```python
from build123d import *

# Parameters (mm, degrees)
F0_R     = 4
F1_DEPTH = 2.5


with BuildPart() as f1:
    # F0 (on Front) → F1 (new body, symmetric)
    with BuildSketch(Plane.XZ):
        with BuildLine():
            Line((0, 8.455922), (-25, 8.455922))
            ThreePointArc((-25, 8.455922), (-33, 0.455922), (-25, -7.544078))
            Line((-25, -7.544078), (0, -7.544078))
            Line((0, -7.544078), (0, 8.455922))
        make_face()
        with Locations((-25, 0.455922)):
            Circle(F0_R, mode=Mode.SUBTRACT)
    extrude(amount=F1_DEPTH, both=True)

    # F2: F1 across face


with BuildPart() as f1_1:
    add(f1.part)
    add(f1.part.mirror(Plane(origin=(0, 0, 0.455922), x_dir=(0, 1, 0), z_dir=(1, 0, 0))))


solid = f1_1.part
```
Source: CAD feature listing. Evaluate the final solid. Frame: model axes, mm. Round coordinates to 2 decimals unless told otherwise and drop trailing zeros. Loops run counter-clockwise (first coordinate to the right, second up) from the corner with the lowest first, then second, coordinate; pieces in that order, holes last. Notation, with made-up numbers: M 82.25,-23.75 L 130.25,-23.75 A14 cw 130.25,-16.75 Z; hole C 42,87 d1. An arc over 180 degrees is marked long. Put each result on its own line as item: value.
(1) Section B-B, the plane z = 3. Return loops of the section in (x, y).
Solutions:
outline: M -32.58,-2.5 L -28.09,-2.5 L -28.09,2.5 L -32.58,2.5 Z; M -21.91,-2.5 L 21.91,-2.5 L 21.91,2.5 L -21.91,2.5 Z; M 28.09,-2.5 L 32.58,-2.5 L 32.58,2.5 L 28.09,2.5 Z
(2) Section D-D, the plane z = -5.75. Return loops of the section in (x, y), and give its area (3 significant figures).
Solutions:
outline: M -30.05,-2.5 L 30.05,-2.5 L 30.05,2.5 L -30.05,2.5 Z
area: 300 mm²
(3) Section A-A, the plane x = -22.5. Return loops of the section in (y, z).
Solutions:
outline: M -2.5,-7.54 L 2.5,-7.54 L 2.5,-2.67 L -2.5,-2.67 Z; M -2.5,3.58 L 2.5,3.58 L 2.5,8.46 L -2.5,8.46 Z
(4) Section C-C, the plane y = -0.7. Return loops of the section in (x, z), and give its area (3 significant figures).
Solutions:
outline: M -25,-7.54 L 25,-7.54 A8 ccw 25,8.46 L -25,8.46 A8 ccw Z; hole C -25,0.46 d8; hole C 25,0.46 d8
area: 901 mm²
(5) Pull-direction query (Z, two-part tool) for faces 1 (the face through (0, 0, -7.544)), 2 (the face through (0, 0, 8.456)), 3 (the face through (-33, 0, 0.6)), 4 (the face through (-28.174, 0.035, -1.978)); classes: released by +Z, released by -Z, zero draft, split by the parting line, or undercut.
Solutions:
face 1: released by -Z
face 2: released by +Z
face 3: split by the parting line
face 4: undercut
(6) Ray query, line 1 (Z direction, x = -25, y = 1); line 2 (X direction, y = -1.85, z = -2.25); line 3 (X direction, y = 0.4, z = -0.75). Return the intervals inside material, ascending. Write a range as [from, to].
Solutions:
line 1: [-7.54, -3.54], [4.46, 8.46]
line 2: [-32.53, -27.95], [-22.05, 22.05], [27.95, 32.53]
line 3: [-32.91, -28.81], [-21.19, 21.19], [28.81, 32.91]
